Work out the finished part from the listing and answer in its coordinate system (mm). A direction names the side the tool comes from. Give positions to 0.01 mm unless a question says otherwise; leave off trailing zeros. Loops run counter-clockwise (first coordinate to the right, second up) from the corner with the lowest first, then second, coordinate; pieces in that order, holes last. Notation, with made-up numbers: (18.25, 10) - (36.25, 10) arc R17 ccw to (36.25, 34) - close; hole circle Ø4 at (55.5, 14). An arc over 180 degrees is marked (long way). Use one line per item in the form item = value. Start each with the question number.
from build123d import *

# Parameters (mm, degrees)
F0_W     = 36
F0_H     = 36
F0_R     = 1.6
F1_DEPTH = 1.8
F2_R     = 2
F3_W     = 5
F3_H     = 7.5
F4_DEPTH = 2
F5_R     = 0.99999


# Not quite as in the source:
# - a fillet or chamfer is up to 0.001 mm smaller than in the source, because OpenCascade refuses the exact size


with BuildPart() as f1:
    # F0 (on Top) → F1 (new body)
    with BuildSketch(Plane.XY):
        Rectangle(F0_W, F0_H)
        with Locations((-15.25, -15.25)):
            Circle(F0_R, mode=Mode.SUBTRACT)
        with Locations((15.25, -15.25)):
            Circle(F0_R, mode=Mode.SUBTRACT)
        with Locations((-15.25, 15.25)):
            Circle(F0_R, mode=Mode.SUBTRACT)
        with Locations((15.25, 15.25)):
            Circle(F0_R, mode=Mode.SUBTRACT)
    extrude(amount=F1_DEPTH)

    # F2
    f2_edges = [f1.edges().sort_by_distance(p)[0] for p in [
        (-18, -18, 0.9),
        (18, -18, 0.9),
        (18, 18, 0.9),
        (-18, 18, 0.9),
    ]]
    fillet(f2_edges, radius=F2_R)

    # F3 (on face) → F4 (join)
    with BuildSketch(Plane.XY.offset(1.8)):
        with Locations((0, -16.75)):
            Rectangle(F3_W, F3_H)
    extrude(amount=F4_DEPTH)

    # F5 (radius 1 in the source; OpenCascade refuses exactly that, so slightly less here)
    f5_edges = [f1.edges().sort_by_distance(p)[0] for p in [
        (-2.5, -19.25, 1.8),
        (-2.5, -16.75, 3.8),
        (2.5, -16.75, 3.8),
        (2.5, -19.25, 1.8),
    ]]
    fillet(f5_edges, radius=F5_R)


solid = f1.part
1) A tool of negligible diameter and unlimited length cuts with its end or side. For faces 1 (the cylindrical face through (-2.215, -19.232, 2.101)), 2 (the flat face through (0, -13, 3)), 3 (the flat face through (-2.5, -15, 2)), from which of +Z, -Z, +X, -X, +Y, -Y can it reach the whole face along a straight path? Write none if from no direction.
2) A cutting plane is placed at A-A (y = -15.25). Give the vertices of the cut face in (x, z).
3) A cutting plane is placed at C-C (x = -15.25). Give the vertices of the cut face in (y, z), plus the area to 3 significant figures.
4) Determine the mould class of faces 4 (the flat face through (0, -18, 1)), 5 (the cylindrical face through (13.65, -15.18, 0.89)), 6 (the cylindrical face through (2.199, -19.232, 2.085)) for opening direction X: released by +X, released by -X, zero draft, split by the parting line, or undercut.
5) A cutting plane is placed at B-B (z = 1.25). Give the vertices of the cut face in (x, y).
6) Flat-ended cylindrical pins translate along their axes: pin 1 Ø1.9 at (x, y) = (-15.25, 15.25) entering from +Z; pin 2 Ø3.5 at (x, y) = (-15.25, -15.25) entering from +Z; pin 3 Ø1.1 at (y, z) = (-17, 2.5) entering from -X; pin 4 Ø0.8 at (x, y) = (0, -19.5) entering from -Z. Find the tip coordinate at first contact, or state that the pin passes through.
7) Find the intervals of material crossed by probe 1 along Y at (x, z) = (-15.25, 0.8); probe 2 along Y at (x, z) = (16.5, 1.35); probe 3 along Z at (x, y) = (6, 9), in increasing order.
Answer sheet:
q1.face_1 = -Z, -X, -Y
q1.face_2 = +Z, +X, -X, +Y
q1.face_3 = +Z, -X, +Y, -Y
q2.outline = (-18, 0) - (-16.85, 0) - (-16.85, 1.8) - (-18, 1.8) - close; (-13.65, 0) - (13.65, 0) - (13.65, 1.8) - (2.5, 1.8) - (2.5, 2.8) arc R1 ccw to (1.5, 3.8) - (-1.5, 3.8) arc R1 ccw to (-2.5, 2.8) - (-2.5, 1.8) - (-13.65, 1.8) - close; (16.85, 0) - (18, 0) - (18, 1.8) - (16.85, 1.8) - close
q3.outline = (-18, 0) - (-16.85, 0) - (-16.85, 1.8) - (-18, 1.8) - close; (-13.65, 0) - (13.65, 0) - (13.65, 1.8) - (-13.65, 1.8) - close; (16.85, 0) - (18, 0) - (18, 1.8) - (16.85, 1.8) - close
q3.area = 53.3 mm²
q4.face_4 = zero draft
q4.face_5 = undercut
q4.face_6 = released by +X
q5.outline = (-18, -16) arc R2 ccw to (-16, -18) - (16, -18) arc R2 ccw to (18, -16) - (18, 16) arc R2 ccw to (16, 18) - (-16, 18) arc R2 ccw to (-18, 16) - close; hole circle Ø3.2 at (-15.25, -15.25); hole circle Ø3.2 at (-15.25, 15.25); hole circle Ø3.2 at (15.25, -15.25); hole circle Ø3.2 at (15.25, 15.25)
q6.pin_1 = through
q6.pin_2 = 1.8
q6.pin_3 = -2.5
q6.pin_4 = 1.8
q7.probe_1 = -18 to -16.85, -13.65 to 13.65, 16.85 to 18
q7.probe_2 = -17.94 to -16.25, -14.25 to 14.25, 16.25 to 17.94
q7.probe_3 = 0 to 1.8
